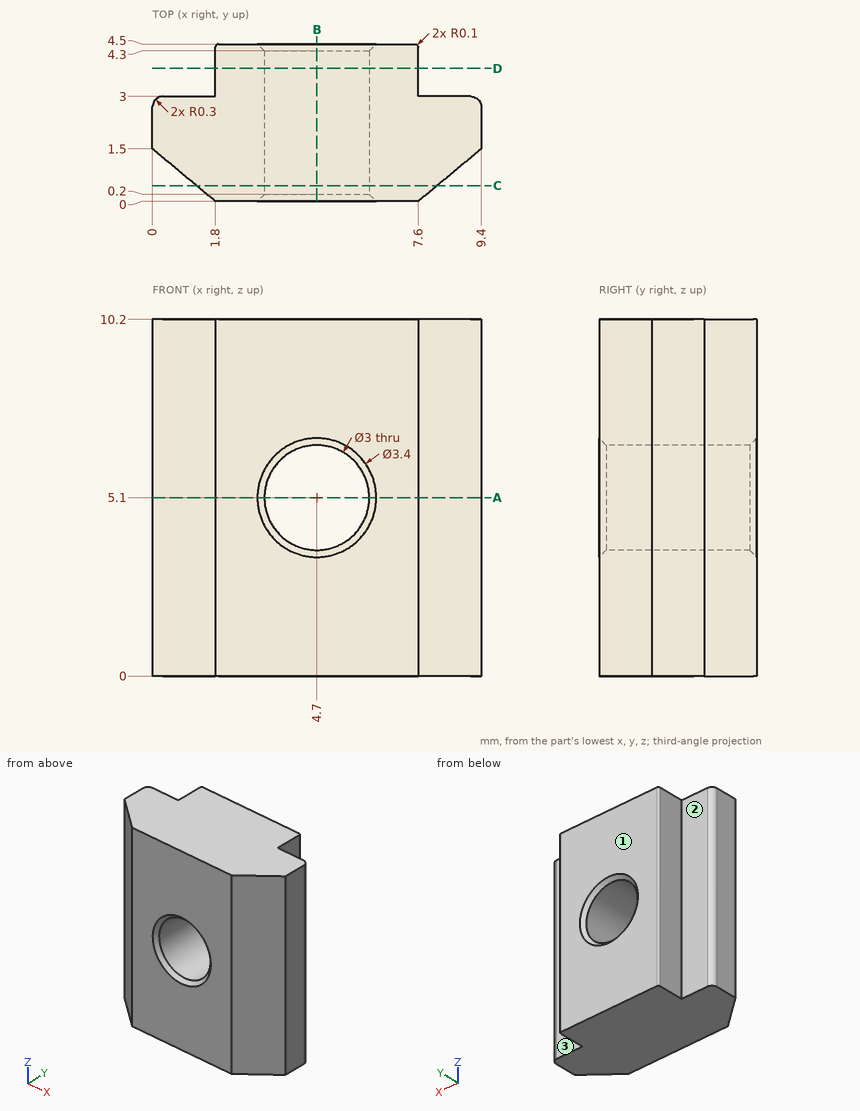
Print and shaded views of the part. All mm, measured from the part's lowest x, y and z. A direction names the side the tool comes from. Round coordinates to 2 decimals unless told otherwise and drop trailing zeros. Order: outer loops, then holes, each group sorted by start corner. A loop starts at its lowest first (then second) coordinate and runs counter-clockwise, first axis right, second up.
Q1. Slice it at B-B (x = 4.7). Write the cut outline in (y, z).
Q2. Which spindle directions (+Z, -Z, +X, -X, +Y, -Y) get a long thin tool onto all of the face, cutting with end or side? Do the marked faces 1, 2 and 3. Say none if no direction does.
Q3. Slice it at A-A (z = 5.1). Write the cut outline in (x, y), and give its area (3 significant figures).
Q4. Slice it at C-C (y = 0.45). Write the cut outline in (x, z).
Q5. Wall check: L1, parallel to X at y = 4, z = 5; L2, parallel to Z at x = 4.75, y = 4.25; L3, parallel to X at y = 1.25, z = 5.1. Give the ranges that are in metal, low to high.
Q6. Drop flat-ended pins along their axis: pin 1 (5 mm diameter, centred on x = 4.7, z = 5.1, fed in from -Y); pin 2 (0.8 mm diameter, centred on x = 1, z = 4.5, fed in from +Y); pin 3 (1.5 mm diameter, centred on y = 4, z = 2.5, fed in from +X); pin 4 (1.5 mm diameter, centred on y = 3.5, z = 4.5, fed in from +X). Give the stop position or say it passes through.
Q7. Slice it at D-D (y = 3.8). Write the cut outline in (x, z), and give its area (3 significant figures).
Results below:
1. outline: (0, 0) - (4.5, 0) - (4.5, 3.4) - (4.3, 3.6) - (0.2, 3.6) - (0, 3.4) - close; (0, 6.8) - (0.2, 6.6) - (4.3, 6.6) - (4.5, 6.8) - (4.5, 10.2) - (0, 10.2) - close
2. face 1: +Z, -Z, +X, -X, +Y
2. face 2: +Z, -Z, -X, +Y
2. face 3: +Z, -Z, +X, +Y
3. outline: (0, 1.5) - (1.8, 0) - (3, 0) - (3.2, 0.2) - (3.2, 4.3) - (3, 4.5) - (1.9, 4.5) arc R0.1 ccw to (1.8, 4.4) - (1.8, 3) - (0.3, 3) arc R0.3 ccw to (0, 2.7) - close; (6.2, 0.2) - (6.4, 0) - (7.6, 0) - (9.4, 1.5) - (9.4, 2.7) arc R0.3 ccw to (9.1, 3) - (7.6, 3) - (7.6, 4.4) arc R0.1 ccw to (7.5, 4.5) - (6.4, 4.5) - (6.2, 4.3) - close
3. area: 20.6 mm2
4. outline: (1.26, 0) - (8.14, 0) - (8.14, 10.2) - (1.26, 10.2) - close; hole circle Ø3 at (4.7, 5.1)
5. L1: x = 1.8 to 3.2, 6.2 to 7.6
5. L2: z = 0 to 3.6, 6.6 to 10.2
5. L3: x = 0.3 to 3.2, 6.2 to 9.1
6. pin 1: stops at y = 0
6. pin 2: stops at y = 3
6. pin 3: stops at x = 7.6
6. pin 4: stops at x = 9.4
7. outline: (1.8, 0) - (7.6, 0) - (7.6, 10.2) - (1.8, 10.2) - close; hole circle Ø3 at (4.7, 5.1)
7. area: 52.1 mm2
